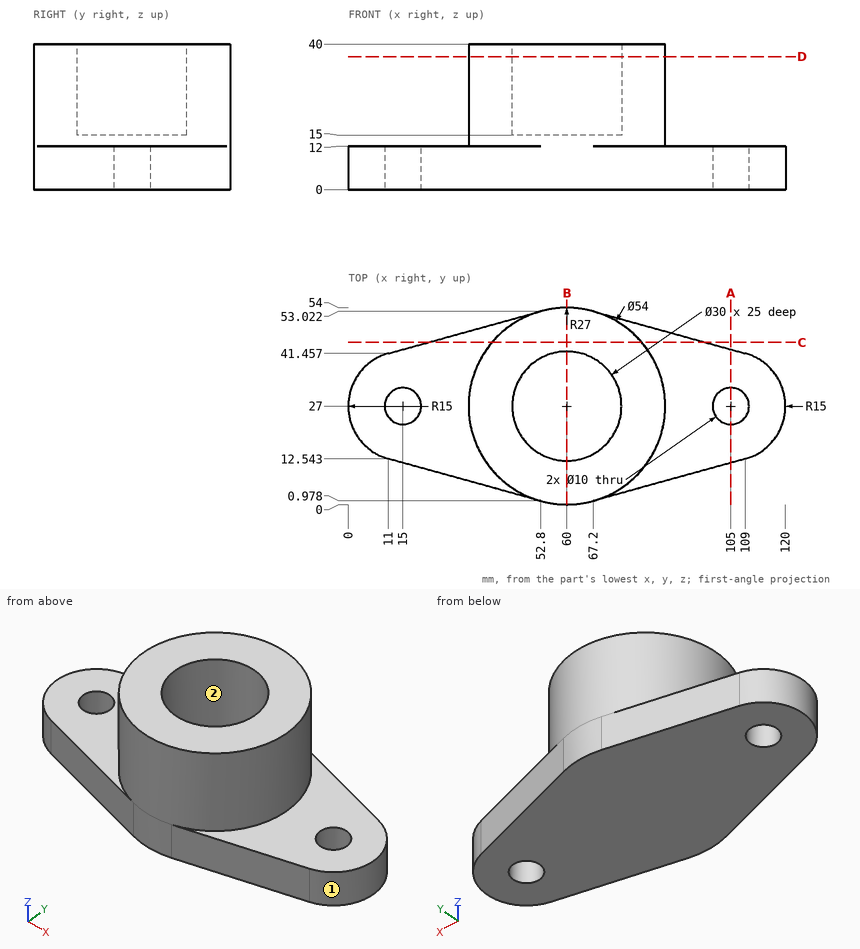
Could you check a few things on this drawing? It's one solid part, dimensions in mm from its lowest x, y, z. A direction names the side the tool comes from. Round coordinates to 2 decimals unless told otherwise and drop trailing zeros. Write each loop counter-clockwise with the first axis right and the second up, starting at its lowest first coordinate (ties: lowest second). Pieces come first, ordered by that corner, then holes. Notation, with made-up numbers: M 59.5,40 L 77.5,40 A28 ccw 77.5,62 Z; hole C 24,23.25 d7. An arc over 180 degrees is marked long. Answer as CSV lines item,"result". Start each with the question number.
1. Suppose I cut it at C-C on y = 44.5. Write out the boundary of the cut face in (x, z), then the cut area to 3 significant figures.
2. Suppose I cut it at B-B on x = 60. Write out the boundary of the cut face in (y, z), then the cut area to 3 significant figures.
3. I need wall thicknesses on probe 1 along Z at (x, y) = (9.5, 17); probe 2 along X at (y, z) = (38, 36); probe 3 along Z at (x, y) = (48.5, 19.5). Which ranges of each line are inside material? Lowest first, please.
4. I'm going to push flat-ended pins straight in: pin 1 Ø12 at (y, z) = (9, 33) entering from +X; pin 2 Ø10 at (y, z) = (24, 33.5) entering from +X; pin 3 Ø1 at (x, y) = (91.5, 12.5) entering from -Z; pin 4 Ø2 at (x, z) = (12.5, 8.5) entering from +Y. Where does each tip first touch, or does it pass through?
5. Suppose I cut it at A-A on x = 105. Write out the boundary of the cut face in (y, z).
6. Suppose I cut it at D-D on z = 36.5. Write out the boundary of the cut face in (x, y), then the cut area to 3 significant figures.
7. On a 3-axis mill with a long thin cutter (end or side, diameter ignored), from which of +Z, -Z, +X, -X, +Y, -Y can I reach the whole of each face in a straight line? I mean the marked faces 1 and 2. Say none if no direction works.
Check result:
1,outline,"M 22,0 L 98,0 L 98,12 L 80.56,12 L 80.56,40 L 39.44,40 L 39.44,12 L 22,12 Z"
1,area,"2,060 mm2"
2,outline,"M 0,0 L 54,0 L 54,40 L 42,40 L 42,15 L 12,15 L 12,40 L 0,40 Z"
2,area,"1,410 mm2"
3,probe 1,"z = 0 to 12"
3,probe 2,"x = 35.34 to 49.8, 70.2 to 84.66"
3,probe 3,"z = 0 to 15"
4,pin 1,"stops at x = 84.19"
4,pin 2,"stops at x = 87"
4,pin 3,"stops at z = 0"
4,pin 4,"stops at y = 42.15"
5,outline,"M 11.44,0 L 22,0 L 22,12 L 11.44,12 Z; M 32,0 L 42.56,0 L 42.56,12 L 32,12 Z"
6,outline,"C 60,27 d54; hole C 60,27 d30"
6,area,"1,580 mm2"
7,face 1,"+Z, -Z, +X"
7,face 2,"+Z"
